Here's how the part is built. I have some questions about the finished solid (model axes, mm). Face numbers are marked on the shaded views. A direction names the side the tool comes from. Coordinates: 2 decimals unless noted, no trailing zeros. Write each loop counter-clockwise with the first axis right and the second up, starting at its lowest first coordinate (ties: lowest second). Pieces come first, ordered by that corner, then holes.
from build123d import *

# Parameters (mm, degrees)
F0_W     = 107.0887371898
F0_H     = 68.4632211924
F2_DEPTH = 12.7
F1_W     = 47.1943685949
F1_H     = 55.7632211924
F3_DEPTH = 20.32
F4_SIZE2 = 5.08
F4_SIZE  = 25.4
F5_R     = 2.54


with BuildPart() as f2:
    # F0 (on Top) → F2 (new body)
    with BuildSketch(Plane.XY):
        Rectangle(F0_W, F0_H)
    extrude(amount=F2_DEPTH)

    # F1 (on Top) → F3 (join)
    with BuildSketch(Plane.XY):
        with Locations((23.5971842974, 0)):
            Rectangle(F1_W, F1_H)
    extrude(amount=F3_DEPTH)

    # F4
    f4_edges = [f2.edges().sort_by_distance(p)[0] for p in [
        (0, 0, 20.32),
    ]]
    f4_side = f2.faces().sort_by_distance((23.597184, 0, 20.32))[0]
    chamfer(f4_edges, length=F4_SIZE, length2=F4_SIZE2, reference=f4_side)

    # F5
    f5_edges = [f2.edges().sort_by_distance(p)[0] for p in [
        (0, 34.231611, 12.7),
        (53.544369, 0, 12.7),
        (0, -34.231611, 12.7),
        (-53.544369, 0, 12.7),
    ]]
    fillet(f5_edges, radius=F5_R)


solid = f2.part
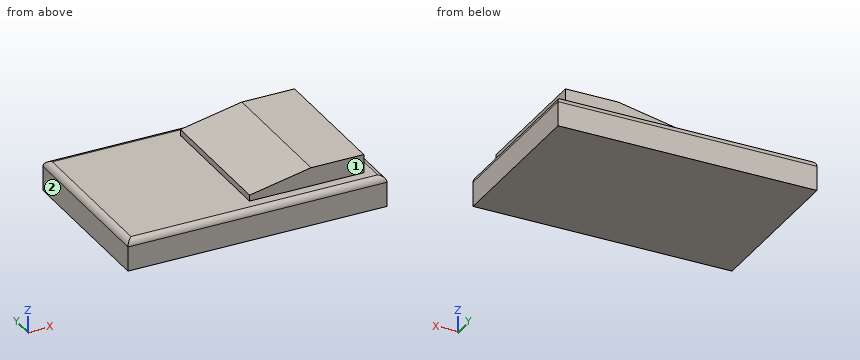
1. For pin 1 Ø6 at (x, y) = (12, -26) entering from +Z; pin 2 Ø4 at (y, z) = (1, 15.5) entering from +X; pin 3 Ø1.3 at (y, z) = (-13.5, 14.5) entering from -X, each with a flat end and sliding along its axis, tell me the tip position at first contact or that it passes through.
2. I want a section at A-A (x = 23.5). List the corners of the cut face in (y, z) for me, then the cut area to 3 significant figures.
3. On a 3-axis mill with a long thin cutter (end or side, diameter ignored), from which of +Z, -Z, +X, -X, +Y, -Y can I reach the whole of each face in a straight line? I mean the marked faces 1 and 2. Say none if no direction works.
4. I want a section at B-B (y = 1.5). List the corners of the cut face in (x, z) for me, then the cut area to 3 significant figures.
5. I want a section at D-D (x = 45). List the corners of the cut face in (y, z) for me.
6. I want a section at C-C (z = 18). List the corners of the cut face in (x, y) for me, then the cut area to 3 significant figures.
7. If I drill on line 1 (Y direction, x = 38.5, z = 15); line 2 (X direction, y = 23, z = 14); line 3 (Z direction, x = -40, y = 21), over which ranges is the centre line in solid material (lowest first)?
Response values:
1. pin 1: stops at z = 18.24
1. pin 2: stops at x = 47.19
1. pin 3: stops at x = 0
2. outline: (-34.23, 0) - (34.23, 0) - (34.23, 10.16) arc R2.54 ccw to (31.69, 12.7) - (27.88, 12.7) - (27.88, 19.94) - (-27.88, 19.94) - (-27.88, 12.7) - (-31.69, 12.7) arc R2.54 ccw to (-34.23, 10.16) - close
2. area: 1,270 mm2
3. face 1: +Z, +X, -X, -Y
3. face 2: +Z, -Z, -X, +Y, -Y
4. outline: (-53.54, 0) - (53.54, 0) - (53.54, 10.16) arc R2.54 ccw to (51, 12.7) - (47.19, 12.7) - (47.19, 20.32) - (25.4, 20.32) - (0, 15.24) - (0, 12.7) - (-51, 12.7) arc R2.54 ccw to (-53.54, 10.16) - close
4. area: 1,650 mm2
5. outline: (-34.23, 0) - (34.23, 0) - (34.23, 10.16) arc R2.54 ccw to (31.69, 12.7) - (27.88, 12.7) - (27.88, 20.32) - (-27.88, 20.32) - (-27.88, 12.7) - (-31.69, 12.7) arc R2.54 ccw to (-34.23, 10.16) - close
6. outline: (13.8, -27.88) - (47.19, -27.88) - (47.19, 27.88) - (13.8, 27.88) - close
6. area: 1,860 mm2
7. line 1: y = -27.88 to 27.88
7. line 2: x = 0 to 47.19
7. line 3: z = 0 to 12.7
